from build123d import *

# Parameters (mm, degrees)
SKETCH1_W           = 140
SKETCH1_H           = 55
BOSS_EXTRUDE1_DEPTH = 35
CUT_EXTRUDE1_DEPTH  = 120
SKETCH4_R           = 26.25
BOSS_EXTRUDE2_DEPTH = 10
SKETCH5_W           = 140
SKETCH5_H           = 20
CUT_EXTRUDE2_DEPTH  = 94.189460294


with BuildPart() as part:
    # Sketch1 → Boss-Extrude1 (new body)
    with BuildSketch(Plane.XY):
        Rectangle(SKETCH1_W, SKETCH1_H)
    extrude(amount=BOSS_EXTRUDE1_DEPTH)

    # Sketch2 → Cut-Extrude1 (cut)
    with BuildSketch(Plane.XY.offset(35)):
        with BuildLine():
            ThreePointArc((70, 0), (60.149153929, -19.600749097), (39.683808374, -27.5))
            Line((39.683808374, -27.5), (70, -27.5))
            Line((70, -27.5), (70, 0))
        make_face()
        with BuildLine():
            Line((-70, -27.5), (-39.683808374, -27.5))
            ThreePointArc((-39.683808374, -27.5), (-60.149153929, -19.600749097), (-70, 0))
            Line((-70, 0), (-70, -27.5))
        make_face()
    extrude(amount=-CUT_EXTRUDE1_DEPTH, mode=Mode.SUBTRACT)

    # Sketch4 → Boss-Extrude2 (add)
    with BuildSketch(Plane(origin=(0, 27.5, 0), x_dir=(1, 0, 0), z_dir=(0, 1, 0))):
        with Locations(Location((0, -18.224998705, 0), (0, 0, 43.97032124))):
            Circle(SKETCH4_R)
    extrude(amount=BOSS_EXTRUDE2_DEPTH)

    # Sketch5 → Cut-Extrude2 (cut, through all)
    with BuildSketch(Plane(origin=(0, 15, 0), x_dir=(1, 0, 0), z_dir=(0, 1, 0))):
        with Locations((0, -17.5)):
            Rectangle(SKETCH5_W, SKETCH5_H)
    extrude(amount=-CUT_EXTRUDE2_DEPTH, mode=Mode.SUBTRACT)


solid = part.part
Build history of the part. All positions in model axes, mm. A direction names the side the tool comes from. Round coordinates to 2 decimals unless told otherwise and drop trailing zeros. Loops run counter-clockwise (first coordinate to the right, second up) from the corner with the lowest first, then second, coordinate; pieces in that order, holes last. Notation, with made-up numbers: (18.5, 70) -> (70.5, 70) arc R29 cw to (70.5, 101) -> close; hole circle Ø2 at (60, -12.5). An arc over 180 degrees is marked (long way). One line per item, written item: value. Start each with the question number.
Q1. Drop flat-ended pins along their axis: pin 1 Ø2 at (x, y) = (-28.5, -20) entering from -Z; pin 2 Ø1.5 at (y, z) = (-4, -0.5) entering from +X; pin 3 Ø1 at (x, y) = (35.5, 22.5) entering from +Z. Give the stop position or say it passes through.
Q2. Cut at A-A on y = 5. List the corners of the cut face in (x, z), plus the area to 3 significant figures.
Q3. Cut at C-C on z = 23.5. List the corners of the cut face in (x, y).
Q4. Cut at D-D on y = 30. List the corners of the cut face in (x, z) (3 decimals).
Q5. Two-plate mould, pull along Z, no slides. Class faces 1 (the face through (-1, 15, 17)), 2 (the face through (60.38, -19.39, 3.8)), 3 (the face through (-1, 0, 0)): released by +Z, released by -Z, zero draft, split by the parting line, or undercut.
Q6. Cut at B-B on x = 0. List the corners of the cut face in (y, z) (3 decimals), plus the area to 3 significant figures.
Q7. Probe line 1 along Z through (x, y) = (35.5, 10.5); line 2 along Y through (x, z) = (-64, 25); line 3 along Y through (x, z) = (-32, 29). List the from-to ranges inside material, lowest first.
Q8. 3-axis set-ups, long thin cutter, end or side, ignore diameter. For faces 4 (the face through (0, 27.5, -3)), 5 (the face through (0, 27.5, 40)), 6 (the face through (-1, -27.5, 31)), 7 (the face through (12.55, 32.43, -4.83)), 8 (the face through (-1, -6, 27.5)): which of +Z, -Z, +X, -X, +Y, -Y reach the whole face in a straight line?
Computed:
1. pin 1: z = 0
1. pin 2: x = 69.46
1. pin 3: z = 35
2. outline: (-70, 0) -> (70, 0) -> (70, 7.5) -> (-70, 7.5) -> close; (-70, 27.5) -> (70, 27.5) -> (70, 35) -> (-70, 35) -> close
2. area: 2,100 mm²
3. outline: (-70, 15) -> (70, 15) -> (70, 27.5) -> (25.71, 27.5) -> (25.71, 37.5) -> (-25.71, 37.5) -> (-25.71, 27.5) -> (-70, 27.5) -> close
4. outline: circle Ø52.5 at (0, 18.225)
5. face 1: undercut
5. face 2: zero draft
5. face 3: released by -Z
6. outline: (-27.5, 0) -> (27.5, 0) -> (27.5, -8.025) -> (37.5, -8.025) -> (37.5, 44.475) -> (27.5, 44.475) -> (27.5, 35) -> (-27.5, 35) -> (-27.5, 27.5) -> (15, 27.5) -> (15, 7.5) -> (-27.5, 7.5) -> close
6. area: 1,600 mm²
7. line 1: 0 to 7.5, 27.5 to 35
7. line 2: 15 to 27.5
7. line 3: -27.5 to 27.5
8. face 4: -Z, +X, -X, -Y
8. face 5: +Z, +X, -X, -Y
8. face 6: +Z, -Z, +X, -X, -Y
8. face 7: +Y
8. face 8: +X, -X, -Y
